Source: CAD feature listing. Evaluate the final solid. Frame: model axes, mm. Coordinates: 2 decimals unless noted, no trailing zeros. Loops run counter-clockwise (first coordinate to the right, second up) from the corner with the lowest first, then second, coordinate; pieces in that order, holes last.
Item 1: Line query: probe 1 along Z at (x, y) = (-105, 4.25); probe 2 along Z at (x, y) = (-94.5, 6.75); probe 3 along X at (y, z) = (6.75, 109). Output: solid intervals per line, ascending.
Item 2: Section query B-B, the plane x = 88. Return the cut outline in (y, z), then the cut area to 4 significant figures.
Item 3: Section query C-C, the plane z = 113.5. Return the cut outline in (x, y).
Item 4: Section query A-A, the plane y = 5.25. Return the cut outline in (x, z), then the cut area to 4 significant figures.
```python
from build123d import *

# Parameters (mm, degrees)
SKETCH1_W           = 310
SKETCH1_H           = 290
BOSS_EXTRUDE1_DEPTH = 10
CUT_EXTRUDE1_DEPTH  = 213.485293609


with BuildPart() as part:
    # Sketch1 → Boss-Extrude1 (new body)
    with BuildSketch(Plane(origin=(0, 0, 0), x_dir=(1, 0, 0), z_dir=(0, 1, 0))):
        Rectangle(SKETCH1_W, SKETCH1_H)
    extrude(amount=BOSS_EXTRUDE1_DEPTH)

    # Sketch2 → Cut-Extrude1 (cut, through all)
    with BuildSketch(Plane(origin=(0, 10, 0), x_dir=(1, 0, 0), z_dir=(0, 1, 0))):
        Polygon((-85.000000005, 145), (-115.000000006, 87.499999999), (-115.000000006, -87.500000001), (-85, -145), (-155, -145), (-155.000000005, 145), align=None)
        Polygon((155, -145), (155.000000005, 145), (85.000000005, 145), (115.000000006, 87.499999999), (115.000000006, -87.500000001), (85, -145), align=None)
    extrude(amount=-CUT_EXTRUDE1_DEPTH, mode=Mode.SUBTRACT)


solid = part.part
```
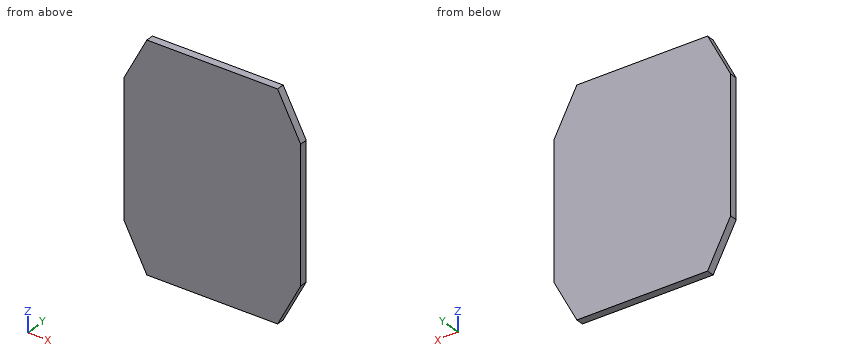
Verdict:
1. probe 1: z = -106.67 to 106.67
1. probe 2: z = -126.79 to 126.79
1. probe 3: x = -103.78 to 103.78
2. outline: (0, -139.25) - (10, -139.25) - (10, 139.25) - (0, 139.25) - close
2. area: 2,785 mm2
3. outline: (-101.43, 0) - (101.43, 0) - (101.43, 10) - (-101.43, 10) - close
4. outline: (-115, -87.5) - (-85, -145) - (85, -145) - (115, -87.5) - (115, 87.5) - (85, 145) - (-85, 145) - (-115, 87.5) - close
4. area: 63,250 mm2
